Source: three-view drawing plus pictorial views. Frame: mm from the lowest corner of the part. Give positions to 0.01 mm unless a question says otherwise; leave off trailing zeros. Loops run counter-clockwise (first coordinate to the right, second up) from the corner with the lowest first, then second, coordinate; pieces in that order, holes last. Notation, with made-up numbers: (-19, 71) -> (19, 71) arc R18 ccw to (19, 86) -> close; hole circle Ø8 at (38.25, -7). An arc over 180 degrees is marked (long way). Answer as a JSON object with one key per item and string values. Group by question number.
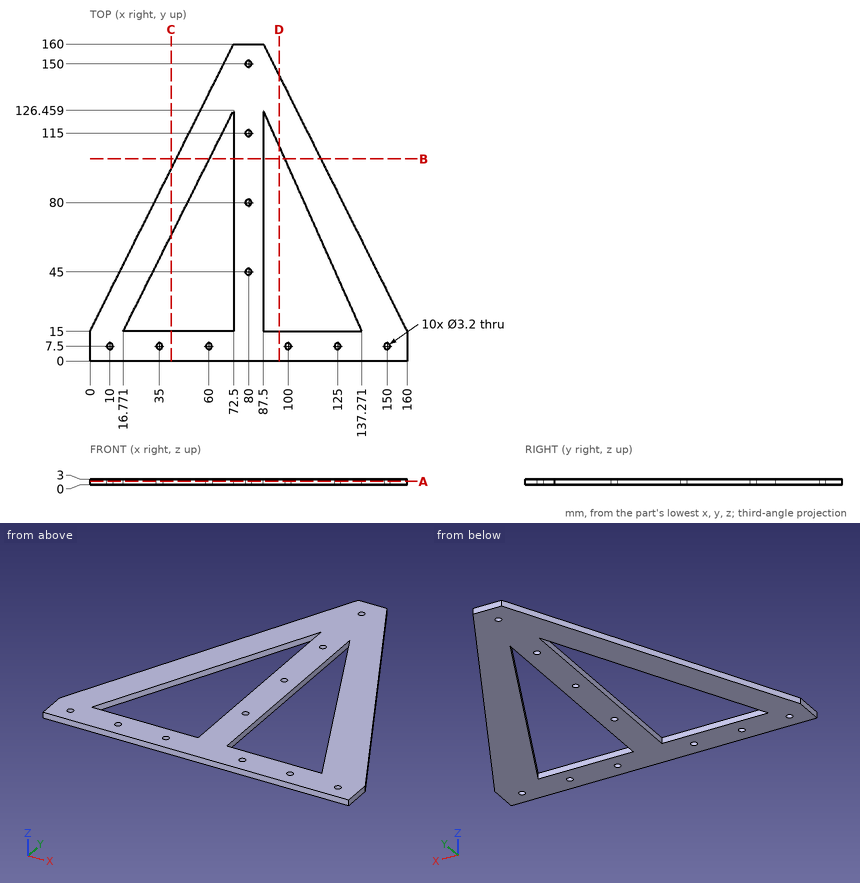
Q1. Section B-B on y = 102. Return the cut outline in (x, z).
Q2. Section A-A on z = 1.8. State how many separate pieces and enclosed holes the cut face has, then the cut area to 3 significant figures.
Q3. Pin query (flat end, axial travel): pin 1 Ø3 at (x, y) = (80, 150) entering from -Z; pin 2 Ø1.5 at (y, z) = (43, 1.5) entering from +X (1 decimal); pin 3 Ø5 at (x, y) = (60, 7.5) entering from -Z; pin 4 Ø1.5 at (x, z) = (48, 1.5) entering from +Y. Return the tip coordinate at first contact, or that it passes through.
Q4. Section D-D on x = 95.5. Return the cut outline in (y, z), then the cut area to 3 significant figures.
Q5. Section C-C on x = 41. Return the cut outline in (y, z).
Q6. Ray query, probe 1 along Y at (x, z) = (80, 2.2); probe 2 along X at (y, z) = (39.5, 2.55); probe 3 along X at (y, z) = (25, 0.55) (1 decimal). Return the intervals inside material, ascending.
Numbers:
{
 "1": {"outline": "(43.5, 0) -> (60.27, 0) -> (60.27, 3) -> (43.5, 3) -> close; (72.5, 0) -> (87.5, 0) -> (87.5, 3) -> (72.5, 3) -> close; (98.42, 0) -> (116.5, 0) -> (116.5, 3) -> (98.42, 3) -> close"},
 "2": {"separate pieces": "1", "enclosed holes": "12", "area": "9,130 mm²"},
 "3": {"pin 1": "passes through", "pin 2": "stops at x = 146.4", "pin 3": "stops at z = 0", "pin 4": "stops at y = 112.5"},
 "4": {"outline": "(0, 0) -> (15, 0) -> (15, 3) -> (0, 3) -> close; (108.54, 0) -> (144, 0) -> (144, 3) -> (108.54, 3) -> close", "area": "151 mm²"},
 "5": {"outline": "(0, 0) -> (15, 0) -> (15, 3) -> (0, 3) -> close; (63.46, 0) -> (97, 0) -> (97, 3) -> (63.46, 3) -> close"},
 "6": {"probe 1": "y = 0 to 43.4, 46.6 to 78.4, 81.6 to 113.4, 116.6 to 148.4, 151.6 to 160", "probe 2": "x = 12.25 to 29.02, 72.5 to 87.5, 126.33 to 147.75", "probe 3": "x = 5 to 21.8, 72.5 to 87.5, 132.8 to 155"}
}
